from build123d import *

# Parameters (mm, degrees)
SKETCH1_R               = 9.525
BASE_EXTRUDE_DEPTH      = 39.6875
CUT_EXTRUDE1_START      = -17.272
CUT_EXTRUDE1_DEPTH      = 17.272
CUT_EXTRUDE2_DEPTH      = 42.911202634
CUT_EXTRUDE2_DEPTH_BACK = 42.911202634
SKETCH3_R               = 3.175
CHAMFER1_SIZE           = 1.27
SKETCH4_R               = 3.175
CUT_EXTRUDE3_DEPTH      = 19.05


with BuildPart() as part:
    # Sketch1 → Base-Extrude (new body)
    with BuildSketch(Plane(origin=(0, 0, 0), x_dir=(0, 0, -1), z_dir=(1, 0, 0))):
        with Locations(Location((0, 0, 0), (0, 0, 180))):
            Circle(SKETCH1_R)
    extrude(amount=BASE_EXTRUDE_DEPTH)

    # Sketch2 → Cut-Extrude1 (cut)
    with BuildSketch(Plane(origin=(39.6875, 0, 0), x_dir=(0, 0, -1), z_dir=(1, 0, 0)).offset(CUT_EXTRUDE1_START)):
        with BuildLine():
            Line((-3.96875, 8.658790241), (-3.96875, -8.658790241))
            ThreePointArc((-3.96875, -8.658790241), (0, -9.525), (3.96875, -8.658790241))
            Line((3.96875, -8.658790241), (3.96875, 8.658790241))
            ThreePointArc((3.96875, 8.658790241), (0, 9.525), (-3.96875, 8.658790241))
        make_face()
    extrude(amount=CUT_EXTRUDE1_DEPTH, mode=Mode.SUBTRACT)

    # Sketch3 → Cut-Extrude2 (cut, two sides: drawn at the far end of the back side and taken through both)
    with BuildSketch(Plane.XY.offset(-CUT_EXTRUDE2_DEPTH_BACK)):
        with Locations((33.274, 0)):
            Circle(SKETCH3_R)
    extrude(amount=CUT_EXTRUDE2_DEPTH + CUT_EXTRUDE2_DEPTH_BACK, mode=Mode.SUBTRACT)

    # Chamfer1
    chamfer1_edges = [part.edges().sort_by_distance(p)[0] for p in [
        (0, 0, -9.525),
        (39.6875, -5.144087929, 8.016482045),
        (39.6875, 0, -9.525),
    ]]
    chamfer(chamfer1_edges, length=CHAMFER1_SIZE)

    # Sketch4 → Cut-Extrude3 (cut)
    with BuildSketch(Plane.ZY):
        Circle(SKETCH4_R)
    extrude(amount=-CUT_EXTRUDE3_DEPTH, mode=Mode.SUBTRACT)


solid = part.part
Design review of the part built by this model. Coordinates are the model's own, in mm. A direction names the side the tool comes from. Round coordinates to 2 decimals unless told otherwise and drop trailing zeros. Write each loop counter-clockwise with the first axis right and the second up, starting at its lowest first coordinate (ties: lowest second). Pieces come first, ordered by that corner, then holes.
Item 1: For faces 1 (the conical face through (39.48, 0.14, 8.46)), 2 (the flat face through (29, 0, 3.969)), list the 3-axis set-ups (+Z, -Z, +X, -X, +Y, -Y) from which the entire face can be reached by the end or side of a thin tool; tool diameter is ignored.
Item 2: Consider section C-C on x = 33.5. Give the boundary of the cut face in (y, z) (3 decimals), and give its area (3 significant figures).
Item 3: Draft analysis for pull direction Z (two halves, no side actions). For faces 3 (the flat face through (0, 4, 0)), 4 (the conical face through (39.48, -0.14, -8.46)), 5 (the flat face through (19.05, 0, 0)), 6 (the cylindrical face through (9.39, -3.1, -0.69)), state which applies: released by +Z, released by -Z, zero draft, split by the parting line, or undercut.
Item 4: For pin 1 Ø2.5 at (y, z) = (-3, -1.5) entering from +X; pin 2 Ø5 at (x, z) = (5.5, -5) entering from +Y; pin 3 Ø8 at (x, z) = (33, 4.5) entering from +Y, all flat-tipped, find the tip position at first contact; note any pin that passes through.
Item 5: Consider section D-D on x = 7. Give the boundary of the cut face in (y, z) (3 decimals), and give its area (3 significant figures).
Item 6: Consider section A-A on y = 0. Count the separate pieces of the cut face and the enclosed holes in it, and give its area (3 significant figures).
Item 7: Wall thickness on L1, parallel to X at y = 0, z = 5.5; L2, parallel to Y at x = 10.5, z = 0 (3 decimals); L3, parallel to X at y = -5.5, z = -0.5: over which ranges is each line inside the solid? List them lowest first.
Check values:
1. face 1: +Z, +X
1. face 2: +X, +Y, -Y
2. outline: (-8.659, -3.969) arc R9.525 ccw to (-3.167, -8.983) - (-3.167, -3.969) - close; (-8.659, 3.969) - (-3.167, 3.969) - (-3.167, 8.983) arc R9.525 ccw to start; (3.167, -8.983) arc R9.525 ccw to (8.659, -3.969) - (3.167, -3.969) - close; (3.167, 3.969) - (8.659, 3.969) arc R9.525 ccw to (3.167, 8.983) - close
2. area: 70.2 mm2
3. face 3: zero draft
3. face 4: released by -Z
3. face 5: undercut
3. face 6: undercut
4. pin 1: stops at x = 22.42
4. pin 2: stops at y = 9.19
4. pin 3: stops at y = 8.66
5. outline: circle Ø19.05 at (0, 0); hole circle Ø6.35 at (0, 0)
5. area: 253 mm2
6. separate pieces: 3
6. enclosed holes: 0
6. area: 424 mm2
7. L1: x = 0 to 30.1, 36.45 to 39.69
7. L2: y = -9.525 to -3.175, 3.175 to 9.525
7. L3: x = 0 to 22.42
